Input: part model. Units: mm. Frame: model coordinates. Round coordinates to 2 decimals unless told otherwise and drop trailing zeros. Loops run counter-clockwise (first coordinate to the right, second up) from the corner with the lowest first, then second, coordinate; pieces in that order, holes last. Notation, with made-up numbers: (42.5, 44.25) -> (67.5, 44.25) arc R12 ccw to (67.5, 53.25) -> close; hole circle Ø8 at (15.25, 69.5). An arc over 180 degrees is marked (long way). Answer as a JSON object with one key per item and string values.
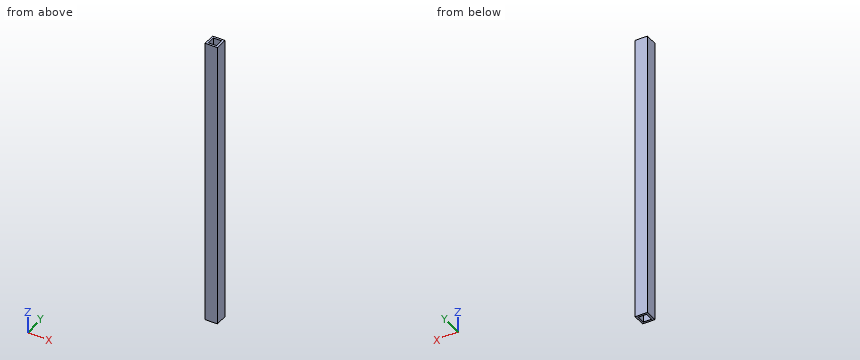
Autodesk Inventor part; units mm, degrees
ref_plane "YZ Plane" through (0, 0, 0) normal (1, 0, 0) x (0, 1, 0)
ref_plane "XZ Plane" through (0, 0, 0) normal (0, 1, 0) x (-1, 0, 0)
ref_plane "XY Plane" through (0, 0, 0) normal (0, 0, 1) x (1, 0, 0)
ref_plane "Work Plane1" through (-350.1142, 119.2278, 28.1686) normal (0, 0, 1) x (0, 1, 0)
sketch "Sketch1" plane through (-350.1142, 119.2278, 28.1686) normal (0, 0, 1) x (0, 1, 0)
  line L0 (70.9812, -246.6013) -> (51.9312, -246.6013)
  line L1 (51.9312, -246.6013) -> (51.9312, -265.6513)
  line L2 (51.9312, -265.6513) -> (70.9812, -265.6513)
  line L3 (70.9812, -265.6513) -> (70.9812, -246.6013)
  line L4 (67.8062, -249.7763) -> (55.1062, -249.7763)
  line L5 (55.1062, -249.7763) -> (55.1062, -262.4763)
  line L6 (55.1062, -262.4763) -> (67.8062, -262.4763)
  line L7 (67.8062, -262.4763) -> (67.8062, -249.7763)
  point P0 (-119.2278, -350.1142)
  dimension "d0" = 19.05
  dimension "d1" = 19.05
  dimension "d2" = 3.175
extrude "Extrusion1" add sketch "Sketch1" along normal blind 457.2
properties part number "StaticForks"
1) Section C-C, the plane z = 163. Output: boundary loops of the cut face in (x, y), plus the area to 3 significant figures.
Output:
{"outline": "(-103.51, 171.16) -> (-84.46, 171.16) -> (-84.46, 190.21) -> (-103.51, 190.21) -> close; hole (-100.34, 174.33) -> (-87.64, 174.33) -> (-87.64, 187.03) -> (-100.34, 187.03) -> close", "area": "202 mm^2"}
2) Ray query, probe 1 along Y at (x, z) = (-95, 199); probe 2 along X at (y, z) = (179.25, 453.5). Return the intervals inside material, ascending.
Output:
{"probe 1": "y = 171.16 to 174.33, 187.03 to 190.21", "probe 2": "x = -103.51 to -100.34, -87.64 to -84.46"}
3) Section B-B, the plane y = 182. Output: boundary loops of the cut face in (x, z).
Output:
{"outline": "(-103.51, 28.17) -> (-100.34, 28.17) -> (-100.34, 485.37) -> (-103.51, 485.37) -> close; (-87.64, 28.17) -> (-84.46, 28.17) -> (-84.46, 485.37) -> (-87.64, 485.37) -> close"}
4) Contact query for a flat-ended pin moving along its axis: P1, Ø6, axis at x = -90.5, y = 184.5, coming from the -Z side. Output: stop coordinate, or through.
Output:
{"P1": "stops at z = 28.17"}
5) Section A-A, the plane x = -92. Output: boundary loops of the cut face in (y, z), plus the area to 3 significant figures.
Output:
{"outline": "(171.16, 28.17) -> (174.33, 28.17) -> (174.33, 485.37) -> (171.16, 485.37) -> close; (187.03, 28.17) -> (190.21, 28.17) -> (190.21, 485.37) -> (187.03, 485.37) -> close", "area": "2,900 mm^2"}
